Job drawing, mm, ordinate dimensions from the low corner. One solid piece. A direction names the side the tool comes from. Give positions to 0.01 mm unless a question says otherwise; leave off trailing zeros. Write each loop counter-clockwise with the first axis right and the second up, starting at its lowest first coordinate (ties: lowest second). Pieces come first, ordered by that corner, then holes. Notation, with made-up numbers: (-27, 5) - (18, 5) arc R25 ccw to (18, 28) - close; hole circle Ø9 at (51, -24.75). An arc over 180 degrees is marked (long way). Answer in a Markdown table with one row per item. Add a question column.
1. Which spindle directions (+Z, -Z, +X, -X, +Y, -Y) get a long thin tool onto all of the face, cutting with end or side? Do the marked faces 4 and 5. Say none if no direction does.
2. Pull direction X, two halves, no side cores. Call the marked faces 1, 2 and 3: released by +X, released by -X, zero draft, split by the parting line, or undercut.
3. Band-saw the part on B-B on z = 4.5. Write the cut outline in (x, y).
4. Band-saw the part on C-C on z = 2.5. Write the cut outline in (x, y), plus the area to 3 significant figures.
5. Probe line 1 along Z through (x, y) = (1.35, 0.4); line 2 along Y through (x, z) = (2.4, 2); line 3 along X through (y, z) = (1.5, 1). List the from-to ranges inside material, lowest first.
6. Band-saw the part on A-A on z = 5.25. Write the cut outline in (x, y), plus the area to 3 significant figures.
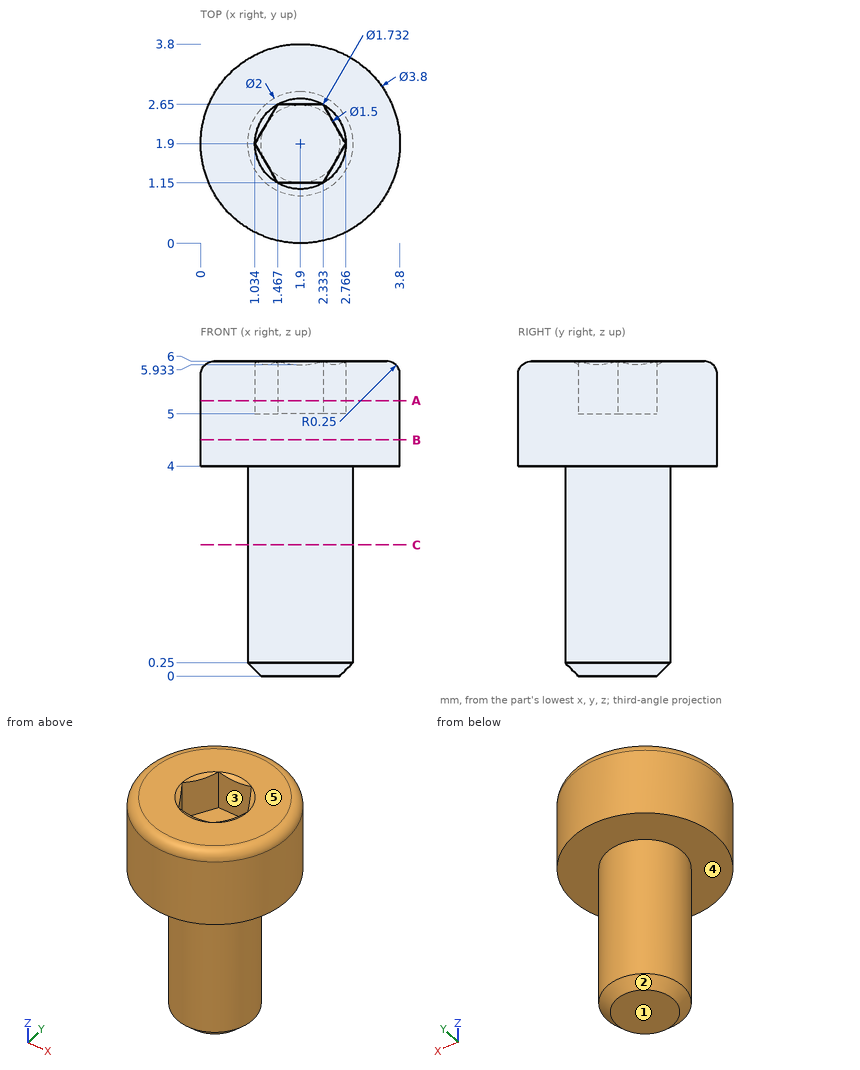
Values:
| question | item | result |
|---|---|---|
| 1 | face 4 | -Z |
| 1 | face 5 | +Z, +X, -X, +Y, -Y |
| 2 | face 1 | zero draft |
| 2 | face 2 | split by the parting line |
| 2 | face 3 | undercut |
| 3 | outline | circle Ø3.8 at (1.9, 1.9) |
| 4 | outline | circle Ø2 at (1.9, 1.9) |
| 4 | area | 3.14 mm² |
| 5 | line 1 | z = 4 to 6 |
| 5 | line 2 | y = 1.03 to 2.77 |
| 5 | line 3 | x = 0.98 to 2.82 |
| 6 | outline | circle Ø3.8 at (1.9, 1.9); hole (1.03, 1.9) - (1.47, 1.15) - (2.33, 1.15) - (2.77, 1.9) - (2.33, 2.65) - (1.47, 2.65) - close |
| 6 | area | 9.39 mm² |
